```python
from build123d import *

# Parameters (mm, degrees)
PAD003_DEPTH  = 3
SKETCH006_W   = 1.8
SKETCH006_H   = 24
SKETCH006_W_2 = 15.6
SKETCH006_H_2 = 1.8
PAD004_DEPTH  = 1.55


with BuildPart() as part:
    # Sketch005 → Pad003 (new body, symmetric)
    with BuildSketch(Plane.XY):
        Polygon((-5, 30.5), (-5, 5), (19.5, 5), (19.5, 10), (0, 10), (0, 30.5), align=None)
    extrude(amount=PAD003_DEPTH, both=True)

    # Sketch006 (on Face8 of Pad003) → Pad004 (join)
    with BuildSketch(Plane.XY.offset(3)):
        with Locations((-2.9, 18.5)):
            Rectangle(SKETCH006_W, SKETCH006_H)
        with Locations((11.7, 7.1)):
            Rectangle(SKETCH006_W_2, SKETCH006_H_2)
    pad004 = extrude(amount=PAD004_DEPTH)

    # Mirrored001: Pad004 across XY
    add(pad004.mirror(Plane.XY))


solid = part.part
```
Geometry: final body of the model. Coordinates: model frame, mm. A direction names the side the tool comes from. Coordinates: 2 decimals unless noted, no trailing zeros. Order: outer loops, then holes, each group sorted by start corner. A loop starts at its lowest first (then second) coordinate and runs counter-clockwise, first axis right, second up. Notation, with made-up numbers: (31, -32) - (81, -32) arc R18 cw to (81, -23) - close; hole circle Ø11 at (67.25, -30). An arc over 180 degrees is marked (long way). Return JSON: item names as keys, results as strings. Group by question number.
1. Cut plane B-B (y = 28.5). Output: boundary loops of the cut face in (x, z).
2. Material intervals for line 1 along Y through (x, z) = (7.5, 0.75); line 2 along X through (y, z) = (11.5, 4.25); line 3 along X through (y, z) = (25, -1.5), sorted ascending. Write a range as [from, to].
3. Cut plane D-D (x = 9.75). Output: boundary loops of the cut face in (y, z), plus the area to 3 significant figures.
4. Cut plane A-A (z = 4.25). Output: boundary loops of the cut face in (x, y).
5. Pin query (flat end, axial travel): pin 1 (0.5 mm diameter, centred on x = 13, z = 4, fed in from +Y); pin 2 (5 mm diameter, centred on x = 8.5, y = 14.5, fed in from +Z); pin 3 (1.2 mm diameter, centred on x = 8.5, z = -3.5, fed in from -Y); pin 4 (4 mm diameter, centred on y = 26, z = 3, fed in from +X). Return the tip coordinate at first contact, or that it passes through.
6. Pull-direction query (X, two-part tool) for faces 1 (the face through (3.9, 7, 4)), 2 (the face through (3.9, 7, -4)), 3 (the face through (-2, 30.5, 0)), 4 (the face through (19.5, 7, 0)); classes: pulls with the +X half, pulls with the -X half, needs draft (parallel to the pull), parting line crosses it, or undercut.
7. Set-up query: faces 5 (the face through (12, 8, -4)), 6 (the face through (12, 8, 4)), 7 (the face through (-3, 6.5, 4)). Return all of +Z, -Z, +X, -X, +Y, -Y with unobstructed straight access to the full face (end or side cutting, diameter ignored); none if empty.
8. Cut plane C-C (z = -1.5). Output: boundary loops of the cut face in (x, y), plus the area to 3 significant figures.
Resolved:
{
 "1": {"outline": "(-5, -3) - (-3.8, -3) - (-3.8, -4.55) - (-2, -4.55) - (-2, -3) - (0, -3) - (0, 3) - (-2, 3) - (-2, 4.55) - (-3.8, 4.55) - (-3.8, 3) - (-5, 3) - close"},
 "2": {"line 1": "y = [5, 10]", "line 2": "x = [-3.8, -2]", "line 3": "x = [-5, 0]"},
 "3": {"outline": "(5, -3) - (6.2, -3) - (6.2, -4.55) - (8, -4.55) - (8, -3) - (10, -3) - (10, 3) - (8, 3) - (8, 4.55) - (6.2, 4.55) - (6.2, 3) - (5, 3) - close", "area": "35.6 mm²"},
 "4": {"outline": "(-3.8, 6.5) - (-2, 6.5) - (-2, 30.5) - (-3.8, 30.5) - close; (3.9, 6.2) - (19.5, 6.2) - (19.5, 8) - (3.9, 8) - close"},
 "5": {"pin 1": "stops at y = 8", "pin 2": "passes through", "pin 3": "stops at y = 5", "pin 4": "stops at x = 0"},
 "6": {"face 1": "undercut", "face 2": "undercut", "face 3": "needs draft", "face 4": "pulls with the +X half"},
 "7": {"face 5": "-Z, +X, +Y", "face 6": "+Z, +X, +Y", "face 7": "+Z, -X, -Y"},
 "8": {"outline": "(-5, 5) - (19.5, 5) - (19.5, 10) - (0, 10) - (0, 30.5) - (-5, 30.5) - close", "area": "225 mm²"}
}
